Autodesk Inventor part; units mm, degrees
ref_plane "YZ Plane" through (0, 0, 0) normal (1, 0, 0) x (0, 1, 0)
ref_plane "XZ Plane" through (0, 0, 0) normal (0, 1, 0) x (-1, 0, 0)
ref_plane "XY Plane" through (0, 0, 0) normal (0, 0, 1) x (1, 0, 0)
sketch "Block1" plane through (0, 0, 0) normal (0, 0, 1) x (1, 0, 0)
  circle A0 centre (74.029, 24.2723) radius 1
  line L0 (49.279, 30.4723) -> (71.779, 30.4723)
  line L1 (71.779, 30.4723) -> (71.779, 18.0723)
  line L2 (71.779, 18.0723) -> (49.279, 18.0723)
  line L3 (49.279, 18.0723) -> (49.279, 30.4723)
  line L4 (49.279, 30.4723) -> (44.779, 30.4723)
  line L5 (44.779, 30.4723) -> (44.779, 18.0723)
  line L6 (44.779, 18.0723) -> (49.279, 18.0723)
  line L7 (49.279, 18.0723) -> (49.279, 30.4723)
  line L8 (71.779, 30.4723) -> (76.279, 30.4723)
  line L9 (76.279, 30.4723) -> (76.279, 18.0723)
  line L10 (76.279, 18.0723) -> (71.779, 18.0723)
  line L11 (71.779, 18.0723) -> (71.779, 30.4723)
  line L12 (44.779, 24.2723) -> (76.279, 24.2723) construction
  line L13 (47.029, 30.4723) -> (47.029, 18.0723) construction
  circle A1 centre (47.029, 24.2723) radius 1
  line L14 (74.029, 30.4723) -> (74.029, 18.0723) construction
  point P0 (60.979, 24.0984)
  dimension "d7" = 22.5
  dimension "d8" = 12.4
  dimension "d9" = 4.5
  dimension "d10" = 4.5
  dimension "d11" = 2
  dimension "d12" = 2
sketch "Sketch1" plane through (0, 0, 0) normal (0, 0, 1) x (1, 0, 0)
  line L0 (-92.7646, -8.503) -> (-89.7646, -8.503)
  line L1 (-89.7646, -8.503) -> (-89.7646, -11.753)
  line L2 (-89.7646, -11.753) -> (-92.7646, -11.753)
  line L3 (-92.7646, -11.753) -> (-92.7646, -8.503)
  line L4 (-92.7646, -21.6527) -> (-89.7646, -21.6527)
  line L5 (-89.7646, -21.6527) -> (-89.7646, -21.7527)
  line L6 (-89.7646, -21.7527) -> (-92.7646, -21.7527)
  line L7 (-92.7646, -21.7527) -> (-92.7646, -21.6527)
  circle A0 centre (0, 0) radius 16.25
  circle A1 centre (0, 13) radius 1
  line L8 (-16.25, 0) -> (16.25, 0) construction
  line L9 (0, 16.25) -> (0, -16.25) construction
  circle A2 centre (0, -13) radius 1
  circle A3 centre (0, 0) radius 3.5
  line L10 (-11.25, 7) -> (-8, 7)
  line L11 (-8, 7) -> (-8, -7)
  line L12 (-8, -7) -> (-11.25, -7)
  line L13 (-11.25, -7) -> (-11.25, 7)
  line L14 (-11.25, 0) -> (-8, 0) construction
  line L15 (11.25, 7) -> (8, 7)
  line L16 (8, 7) -> (8, -7)
  line L17 (8, -7) -> (11.25, -7)
  line L18 (11.25, -7) -> (11.25, 7)
  line L19 (11.25, 0) -> (8, 0) construction
  dimension "d0" = 3
  dimension "mat" = 3.25
  dimension "d2" = 3
  dimension "d3" = 0.1
  dimension "d23" = 32.5
  dimension "d24" = 2
  dimension "d25" = 12
  dimension "d28" = 7
  dimension "d29" = 3.25
  dimension "d30" = 14
  dimension "d31" = 5
extrude "Extrusion3" add sketch "Sketch1" along normal blind 3.25 contours A0
equation "\"d29\" = mat"
equation "\"d32\" = mat"
properties part number "arm-servo"
Part model, mm, in its own coordinate system. A direction names the side the tool comes from. Coordinates: 2 decimals unless noted, no trailing zeros. Write each loop counter-clockwise with the first axis right and the second up, starting at its lowest first coordinate (ties: lowest second). Pieces come first, ordered by that corner, then holes.
Item 1: Slice it at C-C (z = 1.45). Write the cut outline in (x, y), and give its area (3 significant figures).
Item 2: Slice it at D-D (x = 0). Write the cut outline in (y, z), and give its area (3 significant figures).
Item 3: Probe line 1 (Y direction, x = 0, z = 1.95); line 2 (X direction, y = 2, z = 1.9); line 3 (Y direction, x = 9, z = 2.75). List the from-to ranges inside material, lowest first.
Item 4: Pin check, flat tips, straight feed: pin 1 (1 mm diameter, centred on y = 8, z = 0.5, fed in from +X); pin 2 (1.6 mm diameter, centred on x = 9.5, z = 2, fed in from -Y); pin 3 (1 mm diameter, centred on x = 9, z = 2.5, fed in from +Y). Stop position of each tip, or through.
Item 5: Slice it at A-A (y = -4). Write the cut outline in (x, z), and give its area (4 significant figures).
Item 6: Which spindle directions (+Z, -Z, +X, -X, +Y, -Y) get a long thin tool onto all of the face, cutting with end or side? Do faces 4 (the face through (0, 4, 3.25)), 5 (the face through (-10, 7, 2)). Say none if no direction does.
Item 7: Slice it at B-B (y = -13). Write the cut outline in (x, z).
Item 8: Mould opens along X. For faces 1 (the face through (0, 4, 0)), 2 (the face through (15.5, -4.88, 1.6)), 3 (the face through (-11.25, 0, 2)) say: released by +X, released by -X, zero draft, split by the parting line, or undercut.
Results found:
1. outline: circle Ø32.5 at (0, 0); hole (-11.25, -7) - (-8, -7) - (-8, 7) - (-11.25, 7) - close; hole circle Ø7 at (0, 0); hole circle Ø2 at (0, -13); hole circle Ø2 at (0, 13); hole (8, -7) - (11.25, -7) - (11.25, 7) - (8, 7) - close
1. area: 694 mm2
2. outline: (-16.25, 0) - (-14, 0) - (-14, 3.25) - (-16.25, 3.25) - close; (-12, 0) - (-3.5, 0) - (-3.5, 3.25) - (-12, 3.25) - close; (3.5, 0) - (12, 0) - (12, 3.25) - (3.5, 3.25) - close; (14, 0) - (16.25, 0) - (16.25, 3.25) - (14, 3.25) - close
2. area: 69.9 mm2
3. line 1: y = -16.25 to -14, -12 to -3.5, 3.5 to 12, 14 to 16.25
3. line 2: x = -16.13 to -11.25, -8 to -2.87, 2.87 to 8, 11.25 to 16.13
3. line 3: y = -13.53 to -7, 7 to 13.53
4. pin 1: stops at x = 14.42
4. pin 2: stops at y = -13.72
4. pin 3: stops at y = 13.85
5. outline: (-15.75, 0) - (-11.25, 0) - (-11.25, 3.25) - (-15.75, 3.25) - close; (-8, 0) - (8, 0) - (8, 3.25) - (-8, 3.25) - close; (11.25, 0) - (15.75, 0) - (15.75, 3.25) - (11.25, 3.25) - close
5. area: 81.25 mm2
6. face 4: +Z, +X, -X, +Y, -Y
6. face 5: +Z, -Z
7. outline: (-9.75, 0) - (-1, 0) - (-1, 3.25) - (-9.75, 3.25) - close; (1, 0) - (9.75, 0) - (9.75, 3.25) - (1, 3.25) - close
8. face 1: zero draft
8. face 2: split by the parting line
8. face 3: undercut
